Read the model definition and answer for the solid it produces. Units are mm, in the model's axes. Face numbers are marked on the shaded views. A direction names the side the tool comes from. Coordinates: 2 decimals unless noted, no trailing zeros. Loops run counter-clockwise (first coordinate to the right, second up) from the corner with the lowest first, then second, coordinate; pieces in that order, holes last. Notation, with made-up numbers: (-39.75, -8) -> (10.25, -8) arc R31 cw to (10.25, 28) -> close; hole circle Ø4 at (-14, 28.5). An arc over 180 degrees is marked (long way). Answer as a JSON object with one key per item and string values. Group by question number.
1) Consider probe 1 along X at (y, z) = (-6.5, -44.5); probe 2 along Z at (x, y) = (14.5, -12); probe 3 along Y at (x, z) = (1, -46). Determine where each line is inside the solid, lowest interval first. Write a range as [from, to].
2) Section D-D, the plane y = -2 is taken. Give the vertices of the cut face in (x, z), plus the area to 3 significant figures.
3) Section B-B, the plane y = -9.5 is taken. Give the vertices of the cut face in (x, z), plus the area to 3 significant figures.
4) Flat-ended cylindrical pins translate along their axes: P1, Ø10, axis at x = 9, y = 6.5, coming from the +Z side; P2, Ø2, axis at y = 3.5, z = -46.5, coming from the +X side; P3, Ø6, axis at x = 13, y = -8, coming from the +Z side. Find the tip coordinate at first contact, or state that the pin passes through.
5) Section C-C, the plane x = 18.25 is taken. Give the vertices of the cut face in (y, z), plus the area to 3 significant figures.
6) Which of the six approach directions +Z, -Z, +X, -X, +Y, -Y give full straight-line access (tool end or side, diameter ignored) to the marked faces 1 and 2?
7) Determine the mould class of the marked faces 3, 4, 5 and 6 for opening direction X: released by +X, released by -X, zero draft, split by the parting line, or undercut.
8) Section A-A, the plane z = -65.5 is taken. Give the vertices of the cut face in (x, y), plus the area to 3 significant figures.
from build123d import *

# Parameters (mm, degrees)
BASE_FLANGE1_DEPTH  = 20
FILLET1_R           = 3
SKETCH2_W           = 45.198925831
SKETCH2_H           = 23.140478888
BOSS_EXTRUDE1_DEPTH = 19
SKETCH3_W           = 14.337687556
SKETCH3_H           = 41.775325978
CUT_EXTRUDE1_DEPTH  = 26
SKETCH4_R           = 2.315491067
CUT_EXTRUDE2_DEPTH  = 26


# Sheet-metal steps are written as plain solids
with BuildPart() as part:
    # Sketch1 → Base-Flange1 (new body)
    with BuildSketch(Plane(origin=(0, 0, 0), x_dir=(0, 0, -1), z_dir=(1, 0, 0))):
        with BuildLine():
            Line((0, 0), (29.2634, 0))
            ThreePointArc((29.2634, 0), (29.784254855, 0.215745145), (30, 0.7366))
            Line((30, 0.7366), (30, 10))
            Line((30, 10), (33, 10))
            Line((33, 10), (33, 0.7366))
            ThreePointArc((33, 0.7366), (31.905575199, -1.905575199), (29.2634, -3))
            Line((29.2634, -3), (0, -3))
            Line((0, -3), (0, 0))
        make_face()
    extrude(amount=BASE_FLANGE1_DEPTH)

    # Fillet1
    fillet1_edges = [part.edges().sort_by_distance(p)[0] for p in [
        (20, -1.5, 0),
        (20, 10, -31.5),
        (0, -1.5, 0),
        (0, 10, -31.5),
    ]]
    fillet(fillet1_edges, radius=FILLET1_R)

    # Sketch2 → Boss-Extrude1 (add)
    with BuildSketch(Plane.ZY):
        with Locations((-55.599462916, -4.570239444)):
            Rectangle(SKETCH2_W, SKETCH2_H)
    extrude(amount=-BOSS_EXTRUDE1_DEPTH)

    # Sketch3 → Cut-Extrude1 (cut)
    with BuildSketch(Plane(origin=(0, -16.140478888, 0), x_dir=(-1, 0, 0), z_dir=(0, -1, 0))):
        with Locations((-9.603922135, 57.311262842)):
            Rectangle(SKETCH3_W, SKETCH3_H)
    extrude(amount=-CUT_EXTRUDE1_DEPTH, mode=Mode.SUBTRACT)

    # Sketch4 → Cut-Extrude2 (cut)
    with BuildSketch(Plane.ZY):
        with Locations((-39.276024705, -5.060706685)):
            Circle(SKETCH4_R)
    extrude(amount=-CUT_EXTRUDE2_DEPTH, mode=Mode.SUBTRACT)


solid = part.part
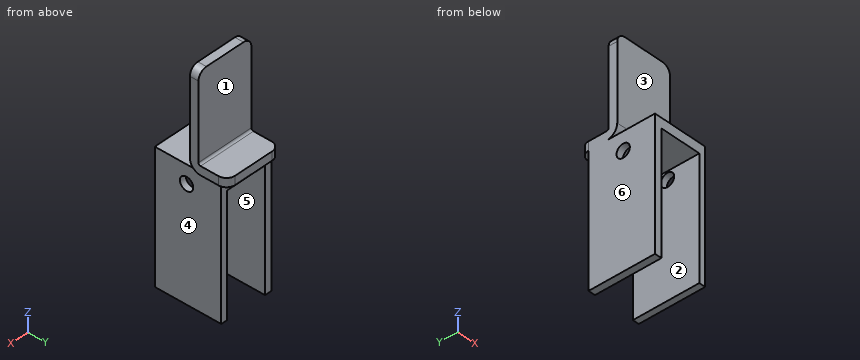
Determined:
{
 "1": {"probe 1": "[0, 2.44], [16.77, 19]", "probe 2": "[-36.42, -33]", "probe 3": "[-16.14, 7]"},
 "2": {"outline": "(0, -78.2) -> (2.44, -78.2) -> (2.44, -36.42) -> (16.77, -36.42) -> (16.77, -78.2) -> (19, -78.2) -> (19, -33) -> (0, -33) -> close; (0, -31.81) -> (20, -31.81) -> (20, -3) arc R3 ccw to (17, 0) -> (3, 0) arc R3 ccw to (0, -3) -> close", "area": "892 mm²"},
 "3": {"outline": "(0, -78.2) -> (2.44, -78.2) -> (2.44, -36.42) -> (16.77, -36.42) -> (16.77, -78.2) -> (19, -78.2) -> (19, -33) -> (0, -33) -> close", "area": "260 mm²"},
 "4": {"P1": "z = -30", "P2": "x = 19", "P3": "z = -33"},
 "5": {"outline": "(-16.14, -78.2) -> (7, -78.2) -> (7, -33) -> (9.73, -33) -> (9.73, -30) -> (0.74, -30) arc R0.74 cw to (0, -29.26) -> (0, -0.27) -> (-3, -0.27) -> (-3, -29.26) arc R3.74 ccw to (0.74, -33) -> (-16.14, -33) -> close; hole circle Ø4.63 at (-5.06, -39.28)", "area": "1,150 mm²"},
 "6": {"face 1": "+Z, +X, -X, +Y", "face 2": "-Z, +Y, -Y"},
 "7": {"face 3": "zero draft", "face 4": "released by +X", "face 5": "undercut", "face 6": "released by -X"},
 "8": {"outline": "(0, -16.14) -> (2.44, -16.14) -> (2.44, 7) -> (0, 7) -> close; (16.77, -16.14) -> (19, -16.14) -> (19, 7) -> (16.77, 7) -> close", "area": "108 mm²"}
}
